```python
from build123d import *

# Parameters (mm, degrees)
SKETCH2_W            = 381
SKETCH2_H            = 127
BOSS_EXTRUDE1_DEPTH  = 6.35
CUT_EXTRUDE3_DEPTH   = 402.659460862
LPATTERN1_COUNT      = 2
LPATTERN1_PITCH      = 50.8
MIRROR1_COPY_1_DEPTH = 402.659460862
SKETCH6_R            = 2.38125
CUT_EXTRUDE4_DEPTH   = 402.659460862
LPATTERN2_COUNT      = 6
LPATTERN2_PITCH      = 63.5
SKETCH7_R            = 2.38125
CUT_EXTRUDE5_DEPTH   = 402.659460862
SKETCH8_W            = 6.35
SKETCH8_H            = 31.75
CUT_EXTRUDE6_DEPTH   = 402.659460862


with BuildPart() as part:
    # Sketch2 → Boss-Extrude1 (new body)
    with BuildSketch(Plane.XY):
        with Locations((190.5, 63.5)):
            Rectangle(SKETCH2_W, SKETCH2_H)
    extrude(amount=BOSS_EXTRUDE1_DEPTH)

    # Sketch5 → Cut-Extrude3 (cut, through all)
    with BuildSketch(Plane(origin=(0, 0, 0), x_dir=(-1, 0, 0), z_dir=(0, 0, -1))):
        Polygon((-381, 101.6), (-381, 82.55), (-374.65, 82.55), (-374.65, 89.535), (-369.951, 89.535), (-369.951, 86.5759), (-366.649, 86.5759), (-366.649, 89.535), (-361.95, 89.535), (-361.95, 94.615), (-366.649, 94.615), (-366.649, 97.5741), (-369.951, 97.5741), (-369.951, 94.615), (-374.65, 94.615), (-374.65, 101.6), align=None)
    cut_extrude3 = extrude(amount=-CUT_EXTRUDE3_DEPTH, mode=Mode.SUBTRACT)

    # LPattern1: Cut-Extrude3 ×2
    with Locations(*[(0, -i * LPATTERN1_PITCH, 0) for i in range(1, LPATTERN1_COUNT)]):
        add(cut_extrude3, mode=Mode.SUBTRACT)

    # Mirror1: Cut-Extrude3 across plane
    add(cut_extrude3.mirror(Plane.ZY.offset(-190.5)), mode=Mode.SUBTRACT)

    # Mirror1 copy 1 sketch → Mirror1 copy 1 (cut, through all)
    with BuildSketch(Plane(origin=(381, -50.8, 0), x_dir=(1, 0, 0), z_dir=(0, 0, -1))):
        Polygon((-381, -101.6), (-381, -82.55), (-374.65, -82.55), (-374.65, -89.535), (-369.951, -89.535), (-369.951, -86.5759), (-366.649, -86.5759), (-366.649, -89.535), (-361.95, -89.535), (-361.95, -94.615), (-366.649, -94.615), (-366.649, -97.5741), (-369.951, -97.5741), (-369.951, -94.615), (-374.65, -94.615), (-374.65, -101.6), align=None)
    extrude(amount=-MIRROR1_COPY_1_DEPTH, mode=Mode.SUBTRACT)

    # Sketch6 → Cut-Extrude4 (cut, through all)
    with BuildSketch(Plane(origin=(0, 0, 0), x_dir=(-1, 0, 0), z_dir=(0, 0, -1))):
        with Locations((-349.25, 121.92)):
            Circle(SKETCH6_R)
    cut_extrude4 = extrude(amount=-CUT_EXTRUDE4_DEPTH, mode=Mode.SUBTRACT)

    # LPattern2: Cut-Extrude4 ×6
    with Locations(*[(-i * LPATTERN2_PITCH, 0, 0) for i in range(1, LPATTERN2_COUNT)]):
        add(cut_extrude4, mode=Mode.SUBTRACT)

    # Sketch7 → Cut-Extrude5 (cut, through all)
    with BuildSketch(Plane(origin=(0, 0, 0), x_dir=(-1, 0, 0), z_dir=(0, 0, -1))):
        with Locations((-369.57, 121.92)):
            Circle(SKETCH7_R)
    cut_extrude5 = extrude(amount=-CUT_EXTRUDE5_DEPTH, mode=Mode.SUBTRACT)

    # Mirror2: Cut-Extrude5 across plane
    add(cut_extrude5.mirror(Plane.ZY.offset(-190.5)), mode=Mode.SUBTRACT)

    # Sketch8 → Cut-Extrude6 (cut, through all)
    with BuildSketch(Plane(origin=(0, 0, 0), x_dir=(-1, 0, 0), z_dir=(0, 0, -1))):
        with Locations((-377.825, 15.875)):
            Rectangle(SKETCH8_W, SKETCH8_H)
    cut_extrude6 = extrude(amount=-CUT_EXTRUDE6_DEPTH, mode=Mode.SUBTRACT)

    # Mirror3: Cut-Extrude6 across plane
    add(cut_extrude6.mirror(Plane.ZY.offset(-190.5)), mode=Mode.SUBTRACT)


solid = part.part
```
Build history of the part. All positions in model axes, mm. A direction names the side the tool comes from. Round coordinates to 2 decimals unless told otherwise and drop trailing zeros.
Item 1: Pin check, flat tips, straight feed: P1, Ø1.5, axis at y = 45.5, z = 3.5, coming from the +X side; P2, Ø2.5, axis at x = 15.5, z = 2, coming from the -Y side; P3, Ø4.5, axis at x = 31.75, y = 121.92, coming from the +Z side; P4, Ø2, axis at y = 92, z = 2.5, coming from the -X side. Stop position of each tip, or through.
Item 2: Saw through at A-A (z = 4). State how many separate pieces and enclosed holes the cut face has, then the cut area to 3 significant figures.
Item 3: Two-plate mould, pull along Y, no slides. Class faces 6 (the face through (188, 64, 0)), 7 (the face through (188, 127, 3)), 8 (the face through (6.35, 98, 3)), 9 (the face through (6.35, 86, 3)): released by +Y, released by -Y, zero draft, split by the parting line, or undercut.
Item 4: Which spindle directions (+Z, -Z, +X, -X, +Y, -Y) get a long thin tool onto all of the face, cutting with end or side? Do faces 1 (the face through (0, 114, 3)), 2 (the face through (6.35, 47, 3)), 3 (the face through (378, 101.6, 3)), 4 (the face through (374.65, 47, 3)), 5 (the face through (3, 101.6, 3)). Say none if no direction does.
Item 5: Drill centre lines: line 1 along Y through (x, z) = (11.43, 2.5); line 2 along Y through (x, z) = (95.25, 5); line 3 along Y through (x, z) = (95.5, 0.75). Where is each one in solid material? Low to high.
Worked answers:
1. P1: stops at x = 374.65
1. P2: stops at y = 0
1. P3: passes through
1. P4: stops at x = 19.05
2. separate pieces: 1
2. enclosed holes: 8
2. area: 47,000 mm2
3. face 6: zero draft
3. face 7: released by +Y
3. face 8: undercut
3. face 9: undercut
4. face 1: +Z, -Z, -X, +Y, -Y
4. face 2: +Z, -Z, -X, -Y
4. face 3: +Z, -Z, +X
4. face 4: +Z, -Z, +X, -Y
4. face 5: +Z, -Z, -X
5. line 1: y = 0 to 35.78, 46.77 to 86.58, 97.57 to 119.54, 124.3 to 127
5. line 2: y = 0 to 119.54, 124.3 to 127
5. line 3: y = 0 to 119.55, 124.29 to 127
